Here's the drawing with two shaded views (mm, measured from the low corner). I have some questions. Round coordinates to 2 decimals unless told otherwise and drop trailing zeros. Order: outer loops, then holes, each group sorted by start corner. A loop starts at its lowest first (then second) coordinate and runs counter-clockwise, first axis right, second up.
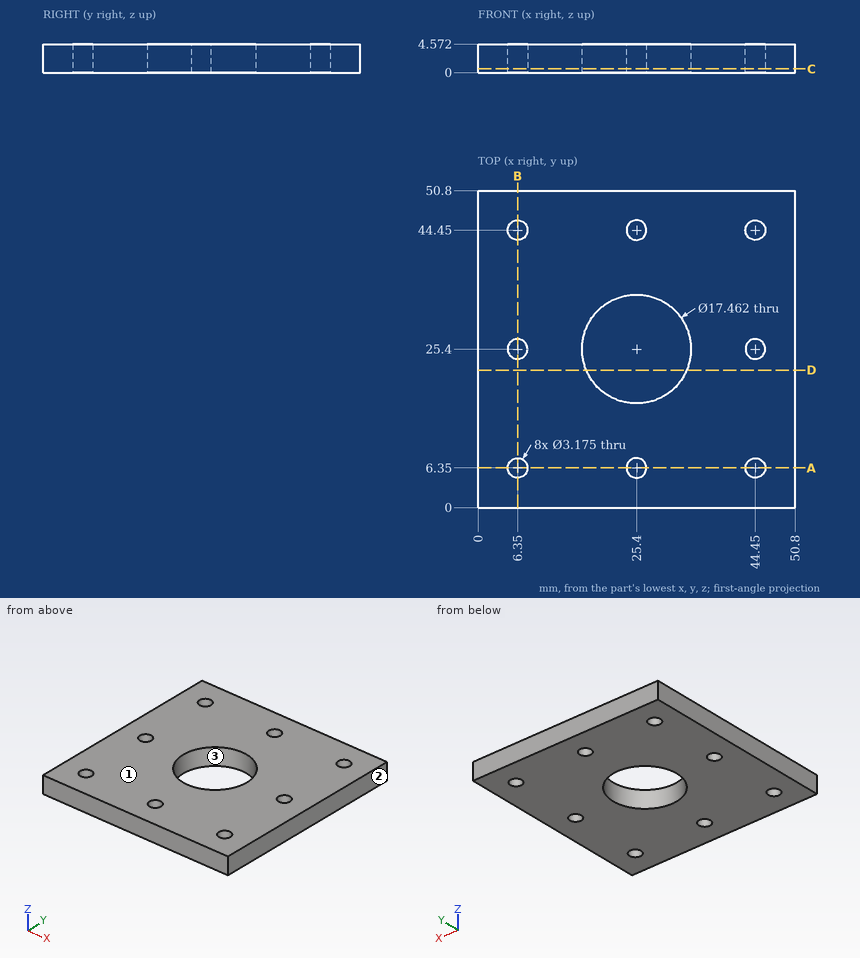
Q1. For P1, Ø3, axis at x = 25.4, y = 6.35, coming from the +Z side, with a flat end and sliding along its axis, tell me the tip position at first contact or that it passes through.
Q2. We'd pull the mould along X, two halves only. Please class the marked faces 1, 2 and 3: released by +X, released by -X, zero draft, split by the parting line, or undercut.
Q3. Imagine slicing it at A-A, the plane y = 6.35. Please give me the cut outline in (x, z).
Q4. Imagine slicing it at D-D, the plane y = 22. Please give me the cut outline in (x, z).
Q5. Imagine slicing it at C-C, the plane z = 0.6. State how many separate pieces and enclosed holes the cut face has, then the cut area to 3 significant figures.
Q6. I need wall thicknesses on L1, parallel to X at y = 25.5, z = 3.85 (1 decimal); L2, parallel to Y at x = 25.4, z = 2.9; L3, parallel to Y at x = 44.45, z = 1.25. Which ranges of each line are inside material? Lowest first, please.
Filled in:
1. P1: passes through
2. face 1: zero draft
2. face 2: released by +X
2. face 3: undercut
3. outline: (0, 0) - (4.76, 0) - (4.76, 4.57) - (0, 4.57) - close; (7.94, 0) - (23.81, 0) - (23.81, 4.57) - (7.94, 4.57) - close; (26.99, 0) - (42.86, 0) - (42.86, 4.57) - (26.99, 4.57) - close; (46.04, 0) - (50.8, 0) - (50.8, 4.57) - (46.04, 4.57) - close
4. outline: (0, 0) - (17.36, 0) - (17.36, 4.57) - (0, 4.57) - close; (33.44, 0) - (50.8, 0) - (50.8, 4.57) - (33.44, 4.57) - close
5. separate pieces: 1
5. enclosed holes: 9
5. area: 2,280 mm2
6. L1: x = 0 to 4.8, 7.9 to 16.7, 34.1 to 42.9, 46 to 50.8
6. L2: y = 0 to 4.76, 7.94 to 16.67, 34.13 to 42.86, 46.04 to 50.8
6. L3: y = 0 to 4.76, 7.94 to 23.81, 26.99 to 42.86, 46.04 to 50.8
